```python
from build123d import *

# Parameters (mm, degrees)
SKETCH1_W          = 12.617819502
SKETCH1_H          = 2
SKETCH1_W_2        = 6.5532
SKETCH1_H_2        = 9.89
SKETCH2_R          = 26.652766262
SKETCH2_R_2        = 14.565
CUT_EXTRUDE1_DEPTH = 10
SKETCH4_R          = 1.0922
CUT_EXTRUDE2_DEPTH = 4.89
CHAMFER1_SIZE      = 0.5
CUT_EXTRUDE3_DEPTH = 10
SKETCH6_W          = 5
SKETCH6_H          = 3.89
CUT_EXTRUDE4_DEPTH = 10


with BuildPart() as part:
    # Sketch1 → Revolve1 (revolve)
    with BuildSketch(Plane(origin=(0, 0, 0), x_dir=(1, 0, 0), z_dir=(0, 1, 0))):
        with Locations((-13.308909751, 3.700473465)):
            Rectangle(SKETCH1_W, SKETCH1_H)
        Polygon((-11.938, 2.700473465), (-19.617819502, 2.700473465), (-19.617819502, 0.700473465), (-13.064619502, 0.700473465), (-11.938, 0.700473465), align=None)
        with Locations((-16.341219502, -4.244526535)):
            Rectangle(SKETCH1_W_2, SKETCH1_H_2)
    revolve(axis=Axis((0, 0, -25.411285606), (0, 0, 1)))

    # Sketch2 → Cut-Extrude1 (cut)
    with BuildSketch(Plane(origin=(0, 0, -4.700473465), x_dir=(-1, 0, 0), z_dir=(0, 0, -1))):
        Circle(SKETCH2_R)
        Circle(SKETCH2_R_2, mode=Mode.SUBTRACT)
    extrude(amount=-CUT_EXTRUDE1_DEPTH, mode=Mode.SUBTRACT)

    # Sketch4 → Cut-Extrude2 (cut, through all)
    with BuildSketch(Plane(origin=(0, 0, 5.299526535), x_dir=(-1, 0, 0), z_dir=(0, 0, -1))):
        with Locations((16.57, 0)):
            Circle(SKETCH4_R)
        with Locations((-16.57, 0)):
            Circle(SKETCH4_R)
    extrude(amount=-CUT_EXTRUDE2_DEPTH, mode=Mode.SUBTRACT)

    # Chamfer1
    chamfer1_edges = [part.edges().sort_by_distance(p)[0] for p in [
        (11.938, 0, -0.700473465),
    ]]
    chamfer(chamfer1_edges, length=CHAMFER1_SIZE)

    # Sketch5 → Cut-Extrude3 (cut)
    with BuildSketch(Plane(origin=(0, 0, 5.299526535), x_dir=(-1, 0, 0), z_dir=(0, 0, -1))):
        with BuildLine():
            Line((0, 19.617819502), (0, 14.565))
            Line((0, 14.565), (2.5, 14.565))
            Line((2.5, 14.565), (2.5, 19.457873522))
            ThreePointArc((2.5, 19.457873522), (1.252555659, 19.577792172), (0, 19.617819502))
        make_face()
        with BuildLine():
            Line((-2.5, 19.457873522), (-2.5, 14.565))
            Line((-2.5, 14.565), (0, 14.565))
            Line((0, 14.565), (0, 19.617819502))
            ThreePointArc((0, 19.617819502), (-1.252555659, 19.577792172), (-2.5, 19.457873522))
        make_face()
    extrude(amount=-CUT_EXTRUDE3_DEPTH, mode=Mode.SUBTRACT)

    # Sketch6 → Cut-Extrude4 (cut)
    with BuildSketch(Plane(origin=(0, 14.565, 0), x_dir=(1, 0, 0), z_dir=(0, 1, 0))):
        with Locations((0, -7.244526535)):
            Rectangle(SKETCH6_W, SKETCH6_H)
    extrude(amount=-CUT_EXTRUDE4_DEPTH, mode=Mode.SUBTRACT)


solid = part.part
```
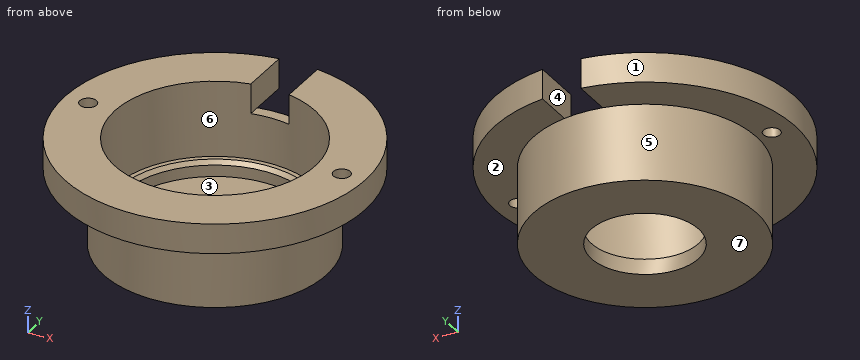
For this review, take the finished solid that the model builds, in its own axes (mm). Face numbers are marked on the shaded views. A direction names the side the tool comes from. Round coordinates to 2 decimals unless told otherwise and drop trailing zeros. Write each loop counter-clockwise with the first axis right and the second up, starting at its lowest first coordinate (ties: lowest second). Pieces come first, ordered by that corner, then holes. Notation, with made-up numbers: (79, 52.25) - (128, 52.25) arc R18 cw to (128, 61.25) - close; hole circle Ø8 at (55.25, 3). An arc over 180 degrees is marked (long way). Answer as a JSON object with one key per item and string values.
1. We need section A-A on x = 0. Give the boundary of the cut face in (y, z) (3 decimals), then the cut area to 3 significant figures.
Response values:
{"outline": "(-19.618, 5.3) - (-14.565, 5.3) - (-14.565, -4.7) - (-7, -4.7) - (-7, -2.7) - (-11.938, -2.7) - (-11.938, -1.2) - (-12.438, -0.7) - (-13.065, -0.7) - (-13.065, 9.19) - (-19.618, 9.19) - close; (7, -4.7) - (14.565, -4.7) - (14.565, 5.3) - (13.065, 5.3) - (13.065, -0.7) - (12.438, -0.7) - (11.938, -1.2) - (11.938, -2.7) - (7, -2.7) - close", "area": "84.0 mm2"}
2. Tool access review of the marked faces 4, 5, 6 and 7: name each direction out of +Z, -Z, +X, -X, +Y, -Y from which nothing blocks a thin tool from reaching the whole face with its end or side.
Response values:
{"face 4": "+Z, +Y", "face 5": "-Z", "face 6": "+Z", "face 7": "-Z, +X, -X, +Y, -Y"}
3. We need section C-C on z = 8. Give the boundary of the cut face in (x, y), then the cut area to 3 significant figures.
Response values:
{"outline": "(-2.5, 12.82) - (-2.5, 19.46) arc R19.62 ccw (long way) to (2.5, 19.46) - (2.5, 12.82) arc R13.06 cw (long way) to start; hole circle Ø2.18 at (-16.57, 0); hole circle Ø2.18 at (16.57, 0)", "area": "632 mm2"}
4. We need section B-B on y = 0. Count the separate pieces of the cut face and the enclosed holes in it, then the cut area to 3 significant figures.
Response values:
{"separate pieces": "4", "enclosed holes": "0", "area": "92.5 mm2"}
5. To check wall thickness, follow line 1 along Y through (x, z) = (0, -3.2) (3 decimals); line 2 along Y through (x, z) = (0, -1.55) (3 decimals). State the ranges of each line that lie inside material, in increasing order.
Response values:
{"line 1": "y = -14.565 to -7, 7 to 14.565", "line 2": "y = -14.565 to -11.938, 11.938 to 14.565"}
6. We need section D-D on x = 16.57. Give the boundary of the cut face in (y, z).
Response values:
{"outline": "(-10.5, 5.3) - (-1.09, 5.3) - (-1.09, 9.19) - (-10.5, 9.19) - close; (1.09, 5.3) - (10.5, 5.3) - (10.5, 9.19) - (1.09, 9.19) - close"}
7. Draft analysis for pull direction Y (two halves, no side actions). For the marked faces 1, 2 and 3, state which applies: +Y half, -Y half, draft (parallel to the pull), parting line (faces both ways), or undercut.
Response values:
{"face 1": "parting line", "face 2": "draft", "face 3": "undercut"}
8. For pin 1 Ø0.9 at (x, y) = (0.5, 14) entering from +Z; pin 2 Ø19 at (x, y) = (0.5, 0.5) entering from +Z; pin 3 Ø6 at (x, z) = (0, 2.5) entering from +Y (3 decimals); pin 4 Ø1.3 at (x, y) = (-16.57, 0) entering from -Z, all flat-tipped, find the tip position at first contact; note any pin that passes through.
Response values:
{"pin 1": "stops at z = 5.3", "pin 2": "stops at z = -2.7", "pin 3": "stops at y = 14.565", "pin 4": "passes through"}
